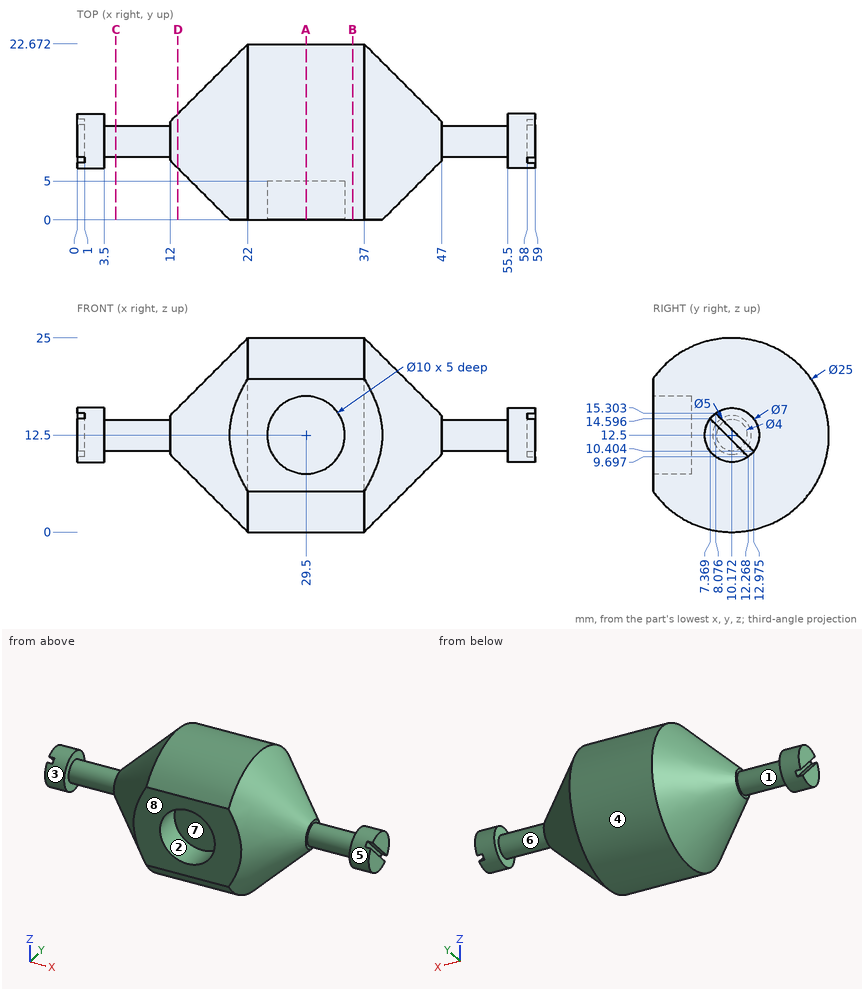
Can you work these out from the drawing? Everything is in mm from the part's minimum corner. A direction names the side the tool comes from. Round coordinates to 2 decimals unless told otherwise and drop trailing zeros. Loops run counter-clockwise (first coordinate to the right, second up) from the corner with the lowest first, then second, coordinate; pieces in that order, holes last. Notation, with made-up numbers: (80, 7.25) - (90, 7.25) arc R9 ccw to (90, 12.25) - close; hole circle Ø5 at (77, -11.5). An arc over 180 degrees is marked (long way). Answer in a Markdown table with one row per item. Add a question column.
(1) If we section it at B-B (x = 35.5): Please give me the cut outline in (y, z) (3 decimals).
(2) For the marked faces 1, 2, 3, 4 and 5, which set-ups out of +Z, -Z, +X, -X, +Y, -Y let a thin tool reach every point of the face, with its end or its side?
(3) If we section it at D-D (x = 13): Please give me the cut outline in (y, z), plus the area to 3 significant figures.
(4) If we section it at C-C (x = 5): Please give me the cut outline in (y, z), plus the area to 3 significant figures.
(5) If we section it at A-A (x = 29.5): Please give me the cut outline in (y, z) (3 decimals).
(6) I'm going to push flat-ended pins straight in: pin 1 (4 mm diameter, centred on y = 4.5, z = 18, fed in from -X); pin 2 (1 mm diameter, centred on x = 22, z = 19, fed in from +Y); pin 3 (3 mm diameter, centred on x = 24, z = 3, fed in from -Y). Where does each tip first touch, or does it pass through?
(7) I need wall thicknesses on line 1 along X through (y, z) = (2, 12.5); line 2 along X through (y, z) = (2.4, 12.5); line 3 along Y through (x, z) = (5.5, 12.5). Which ranges of each line are inside material? Lowest first, please.
(8) If we mould it in two halves opening along X, with no side actions, what happens to the marked faces 6, 7 and 8? For each: pulls with the +X half, pulls with the -X half, needs draft (parallel to the pull), parting line crosses it, or undercut.
Model answer:
| question | item | result |
|---|---|---|
| 1 | outline | (0, 5.235) arc R12.5 ccw (long way) to (0, 19.765) - close |
| 2 | face 1 | none |
| 2 | face 2 | -Y |
| 2 | face 3 | -X |
| 2 | face 4 | +X, -X |
| 2 | face 5 | +X |
| 3 | outline | circle Ø7 at (10.17, 12.5) |
| 3 | area | 38.5 mm² |
| 4 | outline | circle Ø4 at (10.17, 12.5) |
| 4 | area | 12.6 mm² |
| 5 | outline | (0, 5.235) arc R12.5 ccw (long way) to (0, 19.765) - (0, 17.5) - (5, 17.5) - (5, 7.5) - (0, 7.5) - close |
| 6 | pin 1 | stops at x = 15.4 |
| 6 | pin 2 | stops at y = 21.14 |
| 6 | pin 3 | stops at y = 0.57 |
| 7 | line 1 | x = 17.67 to 24.5, 34.5 to 41.33 |
| 7 | line 2 | x = 17.27 to 24.5, 34.5 to 41.73 |
| 7 | line 3 | y = 8.17 to 12.17 |
| 8 | face 6 | undercut |
| 8 | face 7 | undercut |
| 8 | face 8 | needs draft |
